CAD build for the part. Positions are in the model's coordinates, mm. A direction names the side the tool comes from. Coordinates: 2 decimals unless noted, no trailing zeros. Write each loop counter-clockwise with the first axis right and the second up, starting at its lowest first coordinate (ties: lowest second). Pieces come first, ordered by that corner, then holes. Notation, with made-up numbers: (45, 6) - (103, 6) arc R26 ccw to (103, 30) - close; hole circle Ø7 at (47, 12.5). An arc over 180 degrees is marked (long way). One line per question, with ' | ' between items. Start each with the question number.
1. Probe line 1 (Y direction, x = 13.5, z = 19); line 2 (X direction, y = 18.75, z = 6.5); line 3 (Z direction, x = 36, y = 9). List the from-to ranges inside material, lowest first.
2. Band-saw the part on B-B, the plane x = 23.5. Write the cut outline in (y, z), then the cut area to 3 significant figures.
3. Band-saw the part on C-C, the plane y = 21. Give the number of separate pieces and of enclosed holes in the cut face, then the cut area to 3 significant figures.
4. Band-saw the part on D-D, the plane z = 28.5. Write the cut outline in (x, y).
5. Flat gauge pins, fed straight in: P1, Ø6.5, axis at y = 10, z = 7, coming from the -X side; P2, Ø5, axis at y = 21.5, z = 18.5, coming from the +X side; P3, Ø13, axis at x = 10, z = 6.5, coming from the +Y side; P4, Ø1.5, axis at y = 20.5, z = 5.5, coming from the -X side. Where does each tip first touch, or does it go through?
6. Two-plate mould, pull along Y, no slides. Class faces 1 (the flat face through (25, 0, 36)), 2 (the cylindrical face through (35.574, 5.512, 35.597)), 3 (the flat face through (31, 22, 18)): +Y half, -Y half, draft (parallel to the pull), parting line (faces both ways), or undercut.
7. Band-saw the part on A-A, the plane z = 6. Write the cut outline in (x, y).
8. Which spindle directions (+Z, -Z, +X, -X, +Y, -Y) get a long thin tool onto all of the face, cutting with end or side? Do faces 4 (the flat face through (13.4, 4.4, 34.6)), 5 (the flat face through (9, 12, 26)), 6 (the flat face through (6.535, 13.846, 1.69)). Say none if no direction does.
from build123d import *

# Parameters (mm, degrees)
EXTRUDE_1_DEPTH     = 50
CUT_EXTRUDE_1_DEPTH = 67.680295137
EXTRUDE_2_DEPTH     = 22
SKETCH_6_W          = 5
SKETCH_6_H          = 38.291343347
CUT_EXTRUDE_5_DEPTH = 50
SKETCH_8_R          = 2.5
SKETCH_8_R_2        = 1
EXTRUDE_4_DEPTH     = 3
CHAMFER_1_SIZE      = 1.8
CHAMFER_1_SIZE_2    = 3.117691454
SKETCH_9_W          = 10
SKETCH_9_H          = 12
CUT_EXTRUDE_6_DEPTH = 3
SKETCH_10_W         = 12
SKETCH_10_H         = 6
CUT_EXTRUDE_7_DEPTH = 3
FILLET_2_R          = 3
FILLET_3_R          = 3
FILLET_4_R          = 3
CUT_EXTRUDE_8_DEPTH = 1
FILLET_7_R          = 2
SKETCH_12_W         = 5
SKETCH_12_H         = 26.517840655
CUT_EXTRUDE_9_DEPTH = 66.543850106
FILLET_8_R          = 10


with BuildPart() as part:
    # Эскиз2 → Бобышка-Вытянуть1 (new body)
    with BuildSketch(Plane(origin=(0, 0, 0), x_dir=(0, 0, -1), z_dir=(1, 0, 0))):
        Polygon((0, 0), (-22.242640687, 0), (-22.242640687, 3), (-16.242640687, 3), (-24.733307334, 11.490666647), (-34.375121479, 0), (-38.291343347, 0), (-17.389626518, 24.909696123), (-15.091493189, 22.981333294), (-22.797578472, 13.797578472), (-12, 3), (0, 3), align=None)
    extrude(amount=EXTRUDE_1_DEPTH)

    # Эскиз3 → Вырез-Вытянуть1 (cut, through all)
    with BuildSketch(Plane(origin=(0, 3, 0), x_dir=(1, 0, 0), z_dir=(0, 1, 0))):
        Polygon((4, -2.535898385), (1, -4.267949192), (1, -7.732050808), (4, -9.464101615), (7, -7.732050808), (7, -4.267949192), align=None)
        Polygon((46, -2.535898385), (43, -4.267949192), (43, -7.732050808), (46, -9.464101615), (49, -7.732050808), (49, -4.267949192), align=None)
    extrude(amount=-CUT_EXTRUDE_1_DEPTH, mode=Mode.SUBTRACT)

    # Эскиз5 → Бобышка-Вытянуть2 (add)
    # profile 1 of 2: a face of its own
    with BuildSketch(Plane(origin=(0, 3, 0), x_dir=(1, 0, 0), z_dir=(0, 1, 0))):
        Polygon((4, -0.226497308), (-1, -3.113248654), (-1, -8.886751346), (4, -11.773502692), (9, -8.886751346), (9, -3.113248654), align=None)
        Polygon((4, -2.535898385), (1, -4.267949192), (1, -7.732050808), (4, -9.464101615), (7, -7.732050808), (7, -4.267949192), align=None, mode=Mode.SUBTRACT)
    # profile 2 of 2: a face of its own
    with BuildSketch(Plane(origin=(0, 3, 0), x_dir=(1, 0, 0), z_dir=(0, 1, 0))):
        Polygon((46, -0.226497308), (41, -3.113248654), (41, -8.886751346), (46, -11.773502692), (51, -8.886751346), (51, -3.113248654), align=None)
        Polygon((46, -2.535898385), (43, -4.267949192), (43, -7.732050808), (46, -9.464101615), (49, -7.732050808), (49, -4.267949192), align=None, mode=Mode.SUBTRACT)
    extrude(amount=EXTRUDE_2_DEPTH)

    # Эскиз6 → Вырез-Вытянуть5 (cut)
    with BuildSketch(Plane.XZ):
        with Locations((48.5, 19.145671674)):
            Rectangle(SKETCH_6_W, SKETCH_6_H)
        with Locations((1.5, 19.145671674)):
            Rectangle(SKETCH_6_W, SKETCH_6_H)
    extrude(amount=-CUT_EXTRUDE_5_DEPTH, mode=Mode.SUBTRACT)

    # Эскиз8 → Бобышка-Вытянуть4 (add)
    # profile 1 of 4: a face of its own
    with BuildSketch(Plane(origin=(0, 18.854805901, 22.47028267), x_dir=(1, 0, 0), z_dir=(0, 0.6427876096865299, 0.766044443118986))):
        with Locations(Location((36.55, 4.684097832, 0), (0, 0, 90))):
            Circle(SKETCH_8_R)
        with Locations(Location((36.55, 4.684097832, 0), (0, 0, 270))):
            Circle(SKETCH_8_R_2, mode=Mode.SUBTRACT)
    # profile 2 of 4: a face of its own
    with BuildSketch(Plane(origin=(0, 18.854805901, 22.47028267), x_dir=(1, 0, 0), z_dir=(0, 0.6427876096865299, 0.766044443118986))):
        with Locations(Location((13.45, 4.684097832, 0), (0, 0, 90))):
            Circle(SKETCH_8_R)
        with Locations(Location((13.45, 4.684097832, 0), (0, 0, 270))):
            Circle(SKETCH_8_R_2, mode=Mode.SUBTRACT)
    # profile 3 of 4: a face of its own
    with BuildSketch(Plane(origin=(0, 18.854805901, 22.47028267), x_dir=(1, 0, 0), z_dir=(0, 0.6427876096865299, 0.766044443118986))):
        with Locations(Location((13.45, -18.875902168, 0), (0, 0, 90))):
            Circle(SKETCH_8_R)
        with Locations(Location((13.45, -18.875902168, 0), (0, 0, 270))):
            Circle(SKETCH_8_R_2, mode=Mode.SUBTRACT)
    # profile 4 of 4: a face of its own
    with BuildSketch(Plane(origin=(0, 18.854805901, 22.47028267), x_dir=(1, 0, 0), z_dir=(0, 0.6427876096865299, 0.766044443118986))):
        with Locations(Location((36.55, -18.875902168, 0), (0, 0, 90))):
            Circle(SKETCH_8_R)
        with Locations(Location((36.55, -18.875902168, 0), (0, 0, 270))):
            Circle(SKETCH_8_R_2, mode=Mode.SUBTRACT)
    extrude(amount=EXTRUDE_4_DEPTH)

    # Фаска1
    # the kernel refuses this chamfer: 3.117691454, 1.8 mm, written as the material it adds along each edge
    with BuildSketch(Plane(origin=(36.55, 4.395025936, 34.603478705), x_dir=(0, 0.7660444431189859, -0.6427876096865299), z_dir=(1, 0, 0))) as chamfer_1_piece_1_section:
        Polygon((2.5 + CHAMFER_1_SIZE, 0), (2.5, CHAMFER_1_SIZE_2), (2.5, 0), align=None)
    chamfer_1_piece_1 = revolve(axis=Axis((36.55, 4.395025936, 34.603478705), (0, 0.6427876096865299, 0.766044443118986)), mode=Mode.PRIVATE)
    chamfer_1_piece_1 = split(chamfer_1_piece_1, bisect_by=Plane(origin=(36.55, 3.695067891, 39.107035111), z_dir=(0, -0.6427876096865299, -0.766044443118986)), keep=Keep.TOP, mode=Mode.PRIVATE)
    add(chamfer_1_piece_1)
    with BuildSketch(Plane(origin=(13.45, 4.395025936, 34.603478705), x_dir=(0, 0.7660444431189862, -0.6427876096865297), z_dir=(1, 0, 0))) as chamfer_1_piece_2_section:
        Polygon((2.5 + CHAMFER_1_SIZE, 0), (2.5, CHAMFER_1_SIZE_2), (2.5, 0), align=None)
    chamfer_1_piece_2 = revolve(axis=Axis((13.45, 4.395025936, 34.603478705), (0, 0.6427876096865299, 0.766044443118986)), mode=Mode.PRIVATE)
    chamfer_1_piece_2 = split(chamfer_1_piece_2, bisect_by=Plane(origin=(13.45, 3.695067891, 39.107035111), z_dir=(0, -0.6427876096865299, -0.766044443118986)), keep=Keep.TOP, mode=Mode.PRIVATE)
    add(chamfer_1_piece_2)
    with BuildSketch(Plane(origin=(36.55, 22.443033016, 19.459402621), x_dir=(0, 0.7660444431189869, -0.6427876096865287), z_dir=(1, 0, 0))) as chamfer_1_piece_3_section:
        Polygon((2.5 + CHAMFER_1_SIZE, 0), (2.5, CHAMFER_1_SIZE_2), (2.5, 0), align=None)
    chamfer_1_piece_3 = revolve(axis=Axis((36.55, 22.443033016, 19.459402621), (0, 0.6427876096865299, 0.766044443118986)), mode=Mode.PRIVATE)
    chamfer_1_piece_3 = split(chamfer_1_piece_3, bisect_by=Plane(origin=(36.55, 25.826754315, 18.482533914), z_dir=(0, -0.7660444431189845, 0.6427876096865317)), keep=Keep.TOP, mode=Mode.PRIVATE)
    chamfer_1_piece_3 = split(chamfer_1_piece_3, bisect_by=Plane(origin=(36.55, 21.742557786, 23.963392996), z_dir=(0, -0.6427876096865299, -0.766044443118986)), keep=Keep.TOP, mode=Mode.PRIVATE)
    add(chamfer_1_piece_3)
    with BuildSketch(Plane(origin=(13.45, 22.443033016, 19.459402621), x_dir=(0, 0.7660444431189863, -0.6427876096865293), z_dir=(1, 0, 0))) as chamfer_1_piece_4_section:
        Polygon((2.5 + CHAMFER_1_SIZE, 0), (2.5, CHAMFER_1_SIZE_2), (2.5, 0), align=None)
    chamfer_1_piece_4 = revolve(axis=Axis((13.45, 22.443033016, 19.459402621), (0, 0.6427876096865299, 0.766044443118986)), mode=Mode.PRIVATE)
    chamfer_1_piece_4 = split(chamfer_1_piece_4, bisect_by=Plane(origin=(13.45, 25.826754315, 18.482533914), z_dir=(0, -0.7660444431189845, 0.6427876096865317)), keep=Keep.TOP, mode=Mode.PRIVATE)
    chamfer_1_piece_4 = split(chamfer_1_piece_4, bisect_by=Plane(origin=(13.45, 21.742557786, 23.963392996), z_dir=(0, -0.6427876096865299, -0.766044443118986)), keep=Keep.TOP, mode=Mode.PRIVATE)
    add(chamfer_1_piece_4)

    # Эскиз9 → Вырез-Вытянуть6 (cut)
    with BuildSketch(Plane(origin=(0, 3, 0), x_dir=(1, 0, 0), z_dir=(0, 1, 0))):
        with Locations((25, -6)):
            Rectangle(SKETCH_9_W, SKETCH_9_H)
    extrude(amount=-CUT_EXTRUDE_6_DEPTH, mode=Mode.SUBTRACT)

    # Эскиз10 → Вырез-Вытянуть7 (cut)
    with BuildSketch(Plane(origin=(0, 18.854805901, 22.47028267), x_dir=(1, 0, 0), z_dir=(0, 0.6427876096865299, 0.766044443118986))):
        with Locations((25, 4.904097832)):
            Rectangle(SKETCH_10_W, SKETCH_10_H)
    extrude(amount=-CUT_EXTRUDE_7_DEPTH, mode=Mode.SUBTRACT)

    # Скругление2
    fillet_2_edges = [part.edges().sort_by_distance(p)[0] for p in [
        (25, 11.490666647, 24.733307334),
    ]]
    fillet(fillet_2_edges, radius=FILLET_2_R)

    # Скругление3
    # the kernel refuses this fillet: 3 mm, written as the material it adds along each edge
    with BuildSketch(Plane(origin=(4, 3, 16.242640687), x_dir=(0, 0.7071067811865437, 0.7071067811865515), z_dir=(1, 0, 0))) as fillet_3_piece_1:
        with BuildLine():
            CenterArc((6.97317985, 3), FILLET_3_R, 155.530199479, 114.469800521)
            Line((4.242640687, 4.242640687), (4.188029904, 4.267493501))
            ThreePointArc((4.188029904, 4.267493501), (2.078893937, 2.16374675), (-0.042426407, 0.042426407))
            Line((-0.042426407, 0.042426407), (0, -0.06))
            Line((0, -0.06), (6.97317985, -0.06))
            Line((6.97317985, -0.06), (6.97317985, 0))
        make_face()
    extrude(amount=42)

    # Скругление4
    fillet_4_edges = [part.edges().sort_by_distance(p)[0] for p in [
        (25, 13.797578472, 22.797578472),
    ]]
    fillet(fillet_4_edges, radius=FILLET_4_R)

    # Эскиз11 → Вырез-Вытянуть8 (cut)
    with BuildSketch(Plane(origin=(0, 18.854805901, 22.47028267), x_dir=(1, 0, 0), z_dir=(0, 0.6427876096865303, 0.7660444431189857))):
        Polygon((25, -2.436363369), (19.083344336, -15.124672388), (25, -12.613201062), (30.916655664, -15.124672388), align=None)
    extrude(amount=-CUT_EXTRUDE_8_DEPTH, mode=Mode.SUBTRACT)

    # Скругление7
    fillet_7_edges = [part.edges().sort_by_distance(p)[0] for p in [
        (30, 1.5, 0),
        (30, 1.5, 12),
        (20, 1.5, 12),
        (20, 1.5, 0),
    ]]
    fillet(fillet_7_edges, radius=FILLET_7_R)

    # Эскиз12 → Вырез-Вытянуть9 (cut, through all)
    with BuildSketch(Plane.XZ):
        with Locations((6.5, 25.03242302)):
            Rectangle(SKETCH_12_W, SKETCH_12_H)
        with Locations((43.5, 25.03242302)):
            Rectangle(SKETCH_12_W, SKETCH_12_H)
    extrude(amount=-CUT_EXTRUDE_9_DEPTH, mode=Mode.SUBTRACT)

    # Скругление8
    # the kernel refuses this fillet: 10 mm, written as the material it adds along each edge
    with BuildSketch(Plane(origin=(41, 0, 11.773502692), x_dir=(0, 0, 1), z_dir=(0, 1, 0))) as fillet_8_piece_1:
        with BuildLine():
            CenterArc((8.660254038, 10), FILLET_8_R, 210, 60)
            Line((0, 5), (0, 0))
            Line((0, 0), (8.660254038, 0))
        make_face()
    extrude(amount=3)
    with BuildSketch(Plane(origin=(41, 0, 11.773502692), x_dir=(0, 0, 1), z_dir=(0, 1, 0))) as fillet_8_piece_2_section:
        with BuildLine():
            CenterArc((8.660254038, 10), FILLET_8_R, 210, 60)
            Line((0, 5), (0, 0))
            Line((0, 0), (8.660254038, 0))
        make_face()
    fillet_8_piece_2 = extrude(amount=24.650635095, mode=Mode.PRIVATE)
    fillet_8_piece_2 = split(fillet_8_piece_2, bisect_by=Plane(origin=(41.119825884, 8.491267272, 17.491267272), z_dir=(0, -0.7071067811865512, 0.7071067811865439)), keep=Keep.TOP, mode=Mode.PRIVATE)
    fillet_8_piece_2 = fillet_8_piece_2 - Plane(origin=(41.119825884, 5.809462415, 23.294743789), x_dir=(0, 0.7071067811865476, 0.7071067811865476), z_dir=(-1, 0, 0)) * Cylinder(3, 84, mode=Mode.PRIVATE)
    add(fillet_8_piece_2)
    with BuildSketch(Plane(origin=(9, 0, 11.773502692), x_dir=(0, 0, 1), z_dir=(0, 1, 0))) as fillet_8_piece_3:
        with BuildLine():
            CenterArc((8.660254038, -10), FILLET_8_R, 90, 60)
            Line((0, -5), (0, 0))
            Line((0, 0), (8.660254038, 0))
        make_face()
    extrude(amount=3)
    with BuildSketch(Plane(origin=(9, 0, 11.773502692), x_dir=(0, 0, 1), z_dir=(0, 1, 0))) as fillet_8_piece_4_section:
        with BuildLine():
            CenterArc((8.660254038, -10), FILLET_8_R, 90, 60)
            Line((0, -5), (0, 0))
            Line((0, 0), (8.660254038, 0))
        make_face()
    fillet_8_piece_4 = extrude(amount=24.650635095, mode=Mode.PRIVATE)
    fillet_8_piece_4 = split(fillet_8_piece_4, bisect_by=Plane(origin=(8.880174116, 8.491267272, 17.491267272), z_dir=(0, -0.7071067811865512, 0.7071067811865439)), keep=Keep.TOP, mode=Mode.PRIVATE)
    fillet_8_piece_4 = fillet_8_piece_4 - Plane(origin=(8.880174116, 5.809462415, 23.294743789), x_dir=(0, 0.7071067811865476, 0.7071067811865476), z_dir=(-1, 0, 0)) * Cylinder(3, 84, mode=Mode.PRIVATE)
    add(fillet_8_piece_4)


solid = part.part
Filled in:
1) line 1: y = 0 to 10, 18.32 to 22.99, 23.36 to 26.14 | line 2: x = 7 to 9, 41 to 43 | line 3: z = 18 to 22.24, 26.82 to 30.74
2) outline: (0, 12) - (3, 12) - (11.85, 20.85) arc R3 cw to (15.9, 21.03) - (18.39, 18.95) - (20.31, 21.25) - (14.52, 26.1) - (13.88, 25.34) - (8.06, 30.22) - (8.7, 30.99) - (0, 38.29) - (0, 34.38) - (8.98, 26.84) arc R3 cw to (9.18, 22.42) - (7.93, 21.17) arc R3 cw to (3, 22.24) - (0, 22.24) - close | area: 154 mm²
3) separate pieces: 4 | enclosed holes: 0 | area: 157 mm²
4) outline: (9, 7) - (41, 7) - (41, 11.67) - (28.24, 11.67) - (28.79, 10.11) - (21.21, 10.11) - (21.76, 11.67) - (9, 11.67) - close
5) P1: stops at x = 4 | P2: stops at x = 41 | P3: stops at y = 25 | P4: stops at x = 7
6) face 1: -Y half | face 2: undercut | face 3: draft
7) outline: (7, 0) - (20, 0) - (20, 3) - (9, 3) - (9, 25) - (7, 25) - close; (30, 0) - (43, 0) - (43, 25) - (41, 25) - (41, 3) - (30, 3) - close
8) face 4: none | face 5: +Z, -X, +Y | face 6: -Z, +Y
